Verification items for the finished model (mm, model axes). Give positions to 0.01 mm unless a question says otherwise; leave off trailing zeros. Order: outer loops, then holes, each group sorted by start corner. A loop starts at its lowest first (then second) coordinate and runs counter-clockwise, first axis right, second up.
(1) Scan lines: L1, parallel to Y at x = -32, z = 2.45; L2, parallel to Y at x = -22, z = 1.7; L3, parallel to Y at x = -56, z = 2.65. Record each from-to range of solid material in increasing order.
(2) Sectioned sample at B-B on y = 19.5. Record the cut outline in (x, z) (3 decimals).
(3) Sectioned sample at A-A on z = 2.25. Record the cut outline in (x, y) (3 decimals).
(4) Sectioned sample at C-C on y = -12.5. Record the cut outline in (x, z) (3 decimals), plus the area to 3 significant figures.
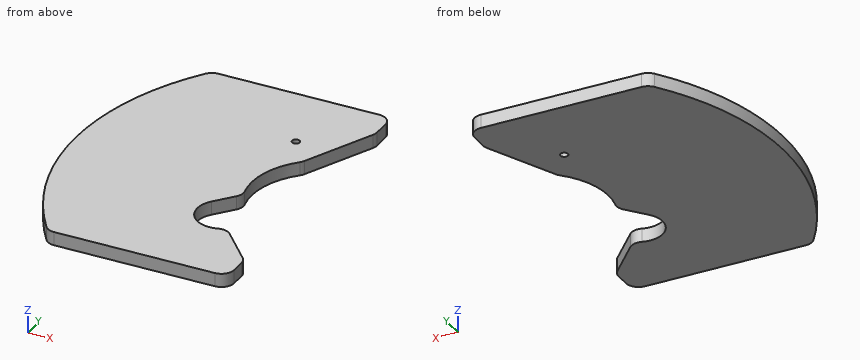
```python
from build123d import *

# Parameters (mm, degrees)
SKETCH1_R           = 0.889
BOSS_EXTRUDE1_DEPTH = 3.175
FILLET1_R           = 3


with BuildPart() as part:
    # Sketch1 → Boss-Extrude1 (new body)
    with BuildSketch(Plane.XY):
        with BuildLine():
            Line((-57.387359122, 37.5), (-15.137359122, 37.5))
            Line((-15.137359122, 37.5), (-15.137359122, 30))
            Line((-15.137359122, 30), (-23.35327626, 12.490642695))
            ThreePointArc((-23.35327626, 12.490642695), (-28.301486723, 4.189647623), (-27.922607376, -5.466840166))
            Line((-27.922607376, -5.466840166), (-32.519153627, -10.979460849))
            ThreePointArc((-32.519153627, -10.979460849), (-32.321991252, -18.88915371), (-24.454232056, -19.726100177))
            Line((-24.454232056, -19.726100177), (-15.137359122, -30))
            Line((-15.137359122, -30), (-15.137359122, -37.5))
            Line((-15.137359122, -37.5), (-57.35903611, -37.5))
            ThreePointArc((-57.35903611, -37.5), (-70.10416265, -0.004807724), (-57.387359122, 37.5))
        make_face()
        with Locations((-28.448323012, 19.5)):
            Circle(SKETCH1_R, mode=Mode.SUBTRACT)
    extrude(amount=BOSS_EXTRUDE1_DEPTH)

    # Fillet1
    fillet1_edges = [part.edges().sort_by_distance(p)[0] for p in [
        (-24.454232056, -19.726100177, 1.5875),
        (-15.137359122, -30, 1.5875),
        (-15.137359122, -37.5, 1.5875),
        (-57.35903611, -37.5, 1.5875),
        (-57.387359122, 37.5, 1.5875),
        (-15.137359122, 37.5, 1.5875),
        (-15.137359122, 30, 1.5875),
        (-23.35327626, 12.490642695, 1.5875),
        (-27.922607376, -5.466840166, 1.5875),
    ]]
    fillet(fillet1_edges, radius=FILLET1_R)


solid = part.part
```
Ans:
1. L1: y = -37.5 to -19.21, -10.36 to 37.5
1. L2: y = -37.5 to -22.43, 15.37 to 37.5
1. L3: y = -37.5 to 37.5
2. outline: (-66.942, 0) - (-29.337, 0) - (-29.337, 3.175) - (-66.942, 3.175) - close; (-27.559, 0) - (-20.064, 0) - (-20.064, 3.175) - (-27.559, 3.175) - close
3. outline: (-58.31, 36.265) arc R61.595 ccw to (-58.282, -36.267) arc R3 ccw to (-55.857, -37.5) - (-18.137, -37.5) arc R3 ccw to (-15.137, -34.5) - (-15.137, -31.158) arc R3 ccw to (-15.915, -29.142) - (-22.954, -21.381) arc R3 ccw to (-26.088, -20.538) arc R6 cw to (-32.519, -10.979) - (-28.944, -6.692) arc R3 ccw to (-28.335, -4.055) arc R16.99 cw to (-23.73, 12.133) arc R3 ccw to (-23.114, 13.001) - (-15.421, 29.394) arc R3 ccw to (-15.137, 30.669) - (-15.137, 34.5) arc R3 ccw to (-18.137, 37.5) - (-55.884, 37.5) arc R3 ccw to start; hole circle Ø1.778 at (-28.448, 19.5)
4. outline: (-68.819, 0) - (-33.443, 0) - (-33.443, 3.175) - (-68.819, 3.175) - close
4. area: 112 mm2
